Verification items for the finished model (mm, model axes). Face numbers are marked on the shaded views. A direction names the side the tool comes from. Give positions to 0.01 mm unless a question says otherwise; leave off trailing zeros. Loops run counter-clockwise (first coordinate to the right, second up) from the corner with the lowest first, then second, coordinate; pieces in that order, holes last. Notation, with made-up numbers: (22, -4) - (60, -4) arc R8 ccw to (60, 9) - close; hole circle Ø4 at (2.5, 25.5). An arc over 180 degrees is marked (long way). One line per item, written item: value. Start each with the question number.
1. Sectioned sample at D-D (y = 8). Record the cut outline in (x, z).
2. Access from +Z, -Z, +X, -X, +Y, -Y to the whole of each face (thin tool, end or side, straight path). Record for the marked faces 3 and 4.
3. Scan lines: L1, parallel to X at y = 5.75, z = 0; L2, parallel to X at y = 7, z = 0. Record each from-to range of solid material in increasing order. Write a range as [from, to].
4. Sectioned sample at A-A (z = 0). Record the cut outline in (x, y).
5. Gauge pin test, flat ends, axial feed: pin 1 (5 mm diameter, centred on x = 11.5, y = 4, fed in from +Z); pin 2 (2 mm diameter, centred on y = 8, z = -11, fed in from +X); pin 3 (1 mm diameter, centred on y = 10, z = 7, fed in from -X). Record the tip position at first contact, or that the pin passes through.
6. Sectioned sample at C-C (x = 34.9). Record the cut outline in (y, z), plus the area to 3 significant figures.
7. Mould release check, pull along Z, two halves, no side actions. Record for the marked faces 1 and 2: pulls with the +Z half, pulls with the -Z half, needs draft (parallel to the pull), parting line crosses it, or undercut.
8. Sectioned sample at B-B (x = 0). Record the cut outline in (y, z).
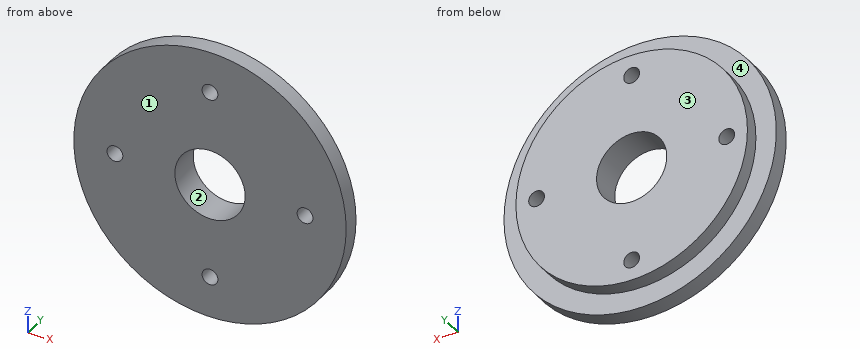
from build123d import *

# Parameters (mm, degrees)
CUT_EXTRUDE1_REACH = 13.35
SKETCH2_R          = 12.9
SKETCH2_R_2        = 2.9


with BuildPart() as part:
    # Sketch1 → Revolve1 (revolve)
    with BuildSketch(Plane.XY):
        Polygon((0, 0), (50, 0), (50, 6.1), (42.5, 6.1), (42.5, 11.35), (0, 11.35), align=None)
    revolve(axis=Axis((0, 0, 0), (0, 1, 0)))

    # Sketch2 → Cut-Extrude1 (cut, up to next)
    with BuildSketch(Plane(origin=(0, 11.35, 0), x_dir=(1, 0, 0), z_dir=(0, 1, 0)), mode=Mode.PRIVATE) as cut_extrude1_sk1:
        Circle(SKETCH2_R)
    cut_extrude1_tool1 = extrude(cut_extrude1_sk1.sketch, amount=-CUT_EXTRUDE1_REACH, mode=Mode.PRIVATE) & part.part
    add(cut_extrude1_tool1.solids().sort_by_distance((0, 11.35, 0))[0], mode=Mode.SUBTRACT)
    # Sketch2 → Cut-Extrude1 (cut, up to next)
    with BuildSketch(Plane(origin=(0, 11.35, 0), x_dir=(1, 0, 0), z_dir=(0, 1, 0)), mode=Mode.PRIVATE) as cut_extrude1_sk2:
        with Locations((0, 34.9)):
            Circle(SKETCH2_R_2)
    cut_extrude1_tool2 = extrude(cut_extrude1_sk2.sketch, amount=-CUT_EXTRUDE1_REACH, mode=Mode.PRIVATE) & part.part
    add(cut_extrude1_tool2.solids().sort_by_distance((0, 11.35, -34.9))[0], mode=Mode.SUBTRACT)
    # Sketch2 → Cut-Extrude1 (cut, up to next)
    with BuildSketch(Plane(origin=(0, 11.35, 0), x_dir=(1, 0, 0), z_dir=(0, 1, 0)), mode=Mode.PRIVATE) as cut_extrude1_sk3:
        with Locations((34.9, 0)):
            Circle(SKETCH2_R_2)
    cut_extrude1_tool3 = extrude(cut_extrude1_sk3.sketch, amount=-CUT_EXTRUDE1_REACH, mode=Mode.PRIVATE) & part.part
    add(cut_extrude1_tool3.solids().sort_by_distance((34.9, 11.35, 0))[0], mode=Mode.SUBTRACT)
    # Sketch2 → Cut-Extrude1 (cut, up to next)
    with BuildSketch(Plane(origin=(0, 11.35, 0), x_dir=(1, 0, 0), z_dir=(0, 1, 0)), mode=Mode.PRIVATE) as cut_extrude1_sk4:
        with Locations((0, -34.9)):
            Circle(SKETCH2_R_2)
    cut_extrude1_tool4 = extrude(cut_extrude1_sk4.sketch, amount=-CUT_EXTRUDE1_REACH, mode=Mode.PRIVATE) & part.part
    add(cut_extrude1_tool4.solids().sort_by_distance((0, 11.35, 34.9))[0], mode=Mode.SUBTRACT)
    # Sketch2 → Cut-Extrude1 (cut, up to next)
    with BuildSketch(Plane(origin=(0, 11.35, 0), x_dir=(1, 0, 0), z_dir=(0, 1, 0)), mode=Mode.PRIVATE) as cut_extrude1_sk5:
        with Locations((-34.9, 0)):
            Circle(SKETCH2_R_2)
    cut_extrude1_tool5 = extrude(cut_extrude1_sk5.sketch, amount=-CUT_EXTRUDE1_REACH, mode=Mode.PRIVATE) & part.part
    add(cut_extrude1_tool5.solids().sort_by_distance((-34.9, 11.35, 0))[0], mode=Mode.SUBTRACT)


solid = part.part
Results are:
1. outline: circle Ø85 at (0, 0); hole circle Ø5.8 at (-34.9, 0); hole circle Ø25.8 at (0, 0); hole circle Ø5.8 at (0, -34.9); hole circle Ø5.8 at (0, 34.9); hole circle Ø5.8 at (34.9, 0)
2. face 3: +Z, -Z, +X, -X, +Y
2. face 4: +Y
3. L1: x = [-50, -37.8], [-32, -12.9], [12.9, 32], [37.8, 50]
3. L2: x = [-42.5, -37.8], [-32, -12.9], [12.9, 32], [37.8, 42.5]
4. outline: (-50, 0) - (-37.8, 0) - (-37.8, 11.35) - (-42.5, 11.35) - (-42.5, 6.1) - (-50, 6.1) - close; (-32, 0) - (-12.9, 0) - (-12.9, 11.35) - (-32, 11.35) - close; (12.9, 0) - (32, 0) - (32, 11.35) - (12.9, 11.35) - close; (37.8, 0) - (50, 0) - (50, 6.1) - (42.5, 6.1) - (42.5, 11.35) - (37.8, 11.35) - close
5. pin 1: stops at z = 49.18
5. pin 2: stops at x = 41.31
5. pin 3: stops at x = -42
6. outline: (0, -35.8) - (6.1, -35.8) - (6.1, -24.25) - (11.35, -24.25) - (11.35, -2.9) - (0, -2.9) - close; (0, 2.9) - (11.35, 2.9) - (11.35, 24.25) - (6.1, 24.25) - (6.1, 35.8) - (0, 35.8) - close
6. area: 626 mm^2
7. face 1: needs draft
7. face 2: undercut
8. outline: (0, -50) - (6.1, -50) - (6.1, -42.5) - (11.35, -42.5) - (11.35, -37.8) - (0, -37.8) - close; (0, -32) - (11.35, -32) - (11.35, -12.9) - (0, -12.9) - close; (0, 12.9) - (11.35, 12.9) - (11.35, 32) - (0, 32) - close; (0, 37.8) - (11.35, 37.8) - (11.35, 42.5) - (6.1, 42.5) - (6.1, 50) - (0, 50) - close
